from build123d import *

# Parameters (mm, degrees)
SKETCH1_R           = 85
SKETCH1_R_2         = 3
BOSS_EXTRUDE1_DEPTH = 12
CUT_EXTRUDE1_DEPTH  = 12
CIRPATTERN1_COUNT   = 3


with BuildPart() as part:
    # Sketch1 → Boss-Extrude1 (new body)
    with BuildSketch(Plane.XY):
        Circle(SKETCH1_R)
        Circle(SKETCH1_R_2, mode=Mode.SUBTRACT)
    extrude(amount=BOSS_EXTRUDE1_DEPTH)

    # Sketch2 → Cut-Extrude1 (cut)
    with BuildSketch(Plane.XY.offset(12)):
        with BuildLine():
            Line((-28.722813233, 80), (28.722813233, 80))
            ThreePointArc((28.722813233, 80), (0, 85), (-28.722813233, 80))
        make_face()
    cut_extrude1 = extrude(amount=-CUT_EXTRUDE1_DEPTH, mode=Mode.SUBTRACT)

    # CirPattern1: Cut-Extrude1 ×3 about axis
    cirpattern1_axis = Axis((0, 0, 0), (0, 0, 1))
    for i in range(1, CIRPATTERN1_COUNT):
        add(cut_extrude1.rotate(cirpattern1_axis, i * 360 / CIRPATTERN1_COUNT), mode=Mode.SUBTRACT)


solid = part.part
Can you work these out from the model? Positions are in its coordinate system, mm. Round coordinates to 2 decimals unless told otherwise and drop trailing zeros. Write each loop counter-clockwise with the first axis right and the second up, starting at its lowest first coordinate (ties: lowest second). Pieces come first, ordered by that corner, then holes. Notation, with made-up numbers: (42, 66.5) -> (86, 66.5) arc R18 cw to (86, 84.5) -> close; hole circle Ø7 at (-38, 15). An arc over 180 degrees is marked (long way). Use one line per item in the form item = value. Start each with the question number.
Q1. If I drill on probe 1 along Y at (x, z) = (0, 4); probe 2 along Y at (x, z) = (15, 5.5); probe 3 along Y at (x, z) = (-69.5, 7.5), over which ranges is the centre line in solid material (lowest first)? Write a range as [from, to].
Q2. Imagine slicing it at D-D (y = 52). Please give me the cut outline in (x, z).
Q3. Imagine slicing it at C-C (z = 10). Please give me the cut outline in (x, y).
Q4. Imagine slicing it at A-A (x = 0). Please give me the cut outline in (y, z), then the cut area to 3 significant figures.
Q5. We'd pull the mould along Y, two halves only. Please class faces 1 (the face through (-1, 17, 0)), 2 (the face through (-3, 0, 6)), 3 (the face through (74.03, 41.77, 5.92)): +Y half, -Y half, draft (parallel to the pull), parting line (faces both ways), or undercut.
Q6. I'm going to push flat-ended pins straight in: P1, Ø3, axis at x = 64, z = 4, coming from the +Y side; P2, Ø5, axis at x = -39.5, z = 2.5, coming from the -Y side; P3, Ø4, axis at y = 44.5, z = 5.5, coming from the +X side. Where does each tip first touch, or does it pass through?
Q7. Imagine slicing it at B-B (y = 0). Please give me the cut outline in (x, z), then the cut area to 3 significant figures.
Worked out:
q1.probe_1 = [-85, -3], [3, 80]
q1.probe_2 = [-83.67, 80]
q1.probe_3 = [-39.62, 48.94]
q2.outline = (-67.24, 0) -> (67.24, 0) -> (67.24, 12) -> (-67.24, 12) -> close
q3.outline = (-83.64, -15.13) -> (-54.92, -64.87) arc R85 ccw to (54.92, -64.87) -> (83.64, -15.13) arc R85 ccw to (28.72, 80) -> (-28.72, 80) arc R85 ccw to start; hole circle Ø6 at (0, 0)
q4.outline = (-85, 0) -> (-3, 0) -> (-3, 12) -> (-85, 12) -> close; (3, 0) -> (80, 0) -> (80, 12) -> (3, 12) -> close
q4.area = 1,910 mm^2
q5.face_1 = draft
q5.face_2 = undercut
q5.face_3 = parting line
q6.P1 = 57.61
q6.P2 = -76.52
q6.P3 = 73.61
q7.outline = (-85, 0) -> (-3, 0) -> (-3, 12) -> (-85, 12) -> close; (3, 0) -> (85, 0) -> (85, 12) -> (3, 12) -> close
q7.area = 1,970 mm^2
